For this review, take the finished solid that the model builds, in its own axes (mm). A direction names the side the tool comes from. Round coordinates to 2 decimals unless told otherwise and drop trailing zeros. Loops run counter-clockwise (first coordinate to the right, second up) from the corner with the lowest first, then second, coordinate; pieces in that order, holes last. Notation, with made-up numbers: (-24.75, 22.25) -> (7.25, 22.25) arc R16 cw to (7.25, 51.25) -> close; hole circle Ø7 at (-9.75, -26.75). An arc over 180 degrees is marked (long way). One line per question, with ' | ' between items. Start each with the question number.
1. Draft analysis for pull direction Y (two halves, no side actions). For faces 3 (the face through (45, 27, 0)), 4 (the face through (47.465, 38.783, -4.26)), 5 (the face through (47, 50, 0)), state which applies: pulls with the +Y half, pulls with the -Y half, needs draft (parallel to the pull), parting line crosses it, or undercut.
2. Wall thickness on line 1 along Y through (x, z) = (48.85, -4); line 2 along X through (y, z) = (1.6, -4); line 3 along Z through (x, y) = (13, 3): over which ranges is each line inside the solid? List them lowest first.
3. For pin 1 Ø10.5 at (y, z) = (31, 4) entering from -X; pin 2 Ø10 at (x, z) = (25.5, -7.5) entering from +Y, all flat-tipped, find the tip position at first contact; note any pin that passes through.
4. For faces 1 (the face through (0, 2, 0)), 2 (the face through (22, 5, 0)), list the 3-axis set-ups (+Z, -Z, +X, -X, +Y, -Y) from which the entire face can be reached by the end or side of a thin tool; tool diameter is ignored.
5. Consider section C-C (y = 36.8). Write out the cut boundary in (x, z), and give its area (3 significant figures).
6. Consider section B-B (z = -4). Write out the cut boundary in (x, y), and give its area (3 significant figures).
7. Consider section D-D (z = 9). Write out the cut boundary in (x, y), and give its area (3 significant figures).
8. Consider section A-A (x = 13.2). Write out the cut boundary in (y, z).
Autodesk Inventor part; units mm, degrees
ref_plane "YZ Plane" through (0, 0, 0) normal (1, 0, 0) x (0, 1, 0)
ref_plane "XZ Plane" through (0, 0, 0) normal (0, 1, 0) x (-1, 0, 0)
ref_plane "XY Plane" through (0, 0, 0) normal (0, 0, 1) x (1, 0, 0)
sketch "Sketch1" plane through (0, 0, 0) normal (0, 0, 1) x (1, 0, 0)
  line L0 (0, 5) -> (45, 5)
  line L1 (45, 5) -> (45, 50)
  line L2 (45, 50) -> (50, 50)
  line L3 (50, 50) -> (50, 0)
  line L4 (50, 0) -> (0, 0)
  line L5 (0, 0) -> (0, 5)
  dimension "d0" = 50
  dimension "d1" = 50
  dimension "d2" = 5
  dimension "d3" = 5
extrude "Extrusion1" add sketch "Sketch1" along normal mid plane 35
sketch "Sketch2" plane through (0, 5, 17.5) normal (0, 1, 0) x (1, 0, 0)
  line L0 (45, 35) -> (0, 35)
  line L1 (0, 35) -> (0, 0)
  circle A0 centre (13.2, 21.5) radius 2
  circle A1 centre (32.3, 21.5) radius 2
  point P0 (0, 17.5)
  dimension "d6" = 4
  dimension "d7" = 13.2
  dimension "d8" = 19.1
  dimension "d9" = 13.5
extrude "Extrusion2" cut sketch "Sketch2" against normal through all
sketch "Sketch3" plane through (45, 5, 17.5) normal (-1, 0, 0) x (0, 0, 1)
  line L0 (0, 45) -> (-35, 45)
  line L1 (-35, 45) -> (-35, 0)
  circle A0 centre (-21.5, 31.8) radius 2
  circle A1 centre (-21.5, 12.7) radius 2
  point P0 (-17.5, -5)
  dimension "d12" = 13.2
  dimension "d13" = 19.1
  dimension "d14" = 13.5
  dimension "d15" = 4
extrude "Extrusion3" cut sketch "Sketch3" against normal through all
Answer block:
1) face 3: needs draft | face 4: undercut | face 5: pulls with the +Y half
2) line 1: y = 0 to 15.7, 19.7 to 34.8, 38.8 to 50 | line 2: x = 0 to 11.2, 15.2 to 30.3, 34.3 to 50 | line 3: z = -17.5 to -5.99, -2.01 to 17.5
3) pin 1: stops at x = 45 | pin 2: stops at y = 5
4) face 1: +Z, -Z, -X, +Y, -Y | face 2: +Z, -Z, -X, +Y
5) outline: (45, -17.5) -> (50, -17.5) -> (50, -6) -> (45, -6) -> close; (45, -2) -> (50, -2) -> (50, 17.5) -> (45, 17.5) -> close | area: 155 mm2
6) outline: (0, 0) -> (11.2, 0) -> (11.2, 5) -> (0, 5) -> close; (15.2, 0) -> (30.3, 0) -> (30.3, 5) -> (15.2, 5) -> close; (34.3, 0) -> (50, 0) -> (50, 15.7) -> (45, 15.7) -> (45, 5) -> (34.3, 5) -> close; (45, 19.7) -> (50, 19.7) -> (50, 34.8) -> (45, 34.8) -> close; (45, 38.8) -> (50, 38.8) -> (50, 50) -> (45, 50) -> close | area: 395 mm2
7) outline: (0, 0) -> (50, 0) -> (50, 50) -> (45, 50) -> (45, 5) -> (0, 5) -> close | area: 475 mm2
8) outline: (0, -17.5) -> (5, -17.5) -> (5, -6) -> (0, -6) -> close; (0, -2) -> (5, -2) -> (5, 17.5) -> (0, 17.5) -> close
